Autodesk Inventor part; units mm, degrees
ref_plane "YZ Plane" through (0, 0, 0) normal (1, 0, 0) x (0, 1, 0)
ref_plane "XZ Plane" through (0, 0, 0) normal (0, 1, 0) x (-1, 0, 0)
ref_plane "XY Plane" through (0, 0, 0) normal (0, 0, 1) x (1, 0, 0)
sketch "Sketch3" plane through (0, 0, 0) normal (0, 0, 1) x (1, 0, 0)
  line L0 (26, 0) -> (21.75, 0.3)
  line L1 (26, 0) -> (26, 18)
  line L2 (21.75, 0.3) -> (21.75, 3.3)
  line L3 (21.75, 3.3) -> (15, 3.3)
  line L4 (15, 3.3) -> (15, 18)
  line L5 (15, 18) -> (26, 18)
  line L6 (0, -3.6) -> (0, 21.6)
  point P0 (0, 0)
  dimension "d5" = 26
  dimension "d6" = 21.75
  dimension "d7" = 0.3
  dimension "d8" = 18
  dimension "d9" = 15
  dimension "d10" = 3
revolve "Revolution1" add sketch "Sketch3" angle 360 about axis through (0, -10, 0) along (0, 1, 0)
sketch "Sketch4" plane through (0, 18, 0) normal (0, 1, 0) x (1, 0, 0)
  point P0 (0, 0)
  point P1 (0, 22)
  point P2 (-19.0526, 11)
  point P3 (-19.0526, -11)
  point P4 (0, -22)
  point P5 (19.0526, -11)
  point P6 (19.0526, 11)
  dimension "d12" = 22
  dimension "d15" = 360
hole "Hole1" at (0, 18, -22) at (-19.0526, 18, -11) at (-19.0526, 18, 11) at (0, 18, 22) at (19.0526, 18, 11) at (19.0526, 18, -11) direction (0, -1, 0) diameter 5 end through all both
properties part number "Adapter1"
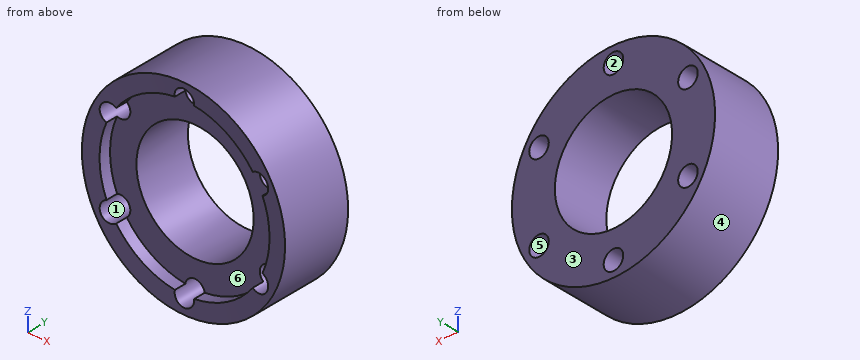
Part model, mm, in its own coordinate system. Face numbers are marked on the shaded views. A direction names the side the tool comes from. Give positions to 0.01 mm unless a question says otherwise; leave off trailing zeros. Order: outer loops, then holes, each group sorted by start corner. A loop starts at its lowest first (then second) coordinate and runs counter-clockwise, first axis right, second up. Notation, with made-up numbers: (-3, 81) - (2, 81) arc R19 cw to (2, 92) - close; hole circle Ø4 at (45, 19.25). An arc over 180 degrees is marked (long way). Use a Markdown table: item, result.
1) Saw through at C-C on x = 0. List the corners of the cut face in (y, z).
Checked values:
| item | result |
|---|---|
| outline | (0, -26) - (18, -26) - (18, -24.5) - (0.11, -24.5) - close; (0, 26) - (0.11, 24.5) - (18, 24.5) - (18, 26) - close; (3.3, -19.5) - (18, -19.5) - (18, -15) - (3.3, -15) - close; (3.3, 15) - (18, 15) - (18, 19.5) - (3.3, 19.5) - close |
2) Saw through at B-B on y = 1.5. List the corners of the cut face in (x, z), plus the area to 3 significant figures.
Checked values:
| item | result |
|---|---|
| outline | circle Ø52 at (0, 0); hole (-19.95, -8.67) arc R2.5 ccw (long way) to (-17.48, -12.94) arc R21.75 ccw to (-2.47, -21.61) arc R2.5 ccw (long way) to (2.47, -21.61) arc R21.75 ccw to (17.48, -12.94) arc R2.5 ccw (long way) to (19.95, -8.67) arc R21.75 ccw to (19.95, 8.67) arc R2.5 ccw (long way) to (17.48, 12.94) arc R21.75 ccw to (2.47, 21.61) arc R2.5 ccw (long way) to (-2.47, 21.61) arc R21.75 ccw to (-17.48, 12.94) arc R2.5 ccw (long way) to (-19.95, 8.67) arc R21.75 ccw to start |
| area | 570 mm² |
3) Saw through at A-A on z = 0. List the corners of the cut face in (x, y), plus the area to 3 significant figures.
Checked values:
| item | result |
|---|---|
| outline | (-26, 0) - (-21.75, 0.3) - (-21.75, 3.3) - (-15, 3.3) - (-15, 18) - (-26, 18) - close; (15, 3.3) - (21.75, 3.3) - (21.75, 0.3) - (26, 0) - (26, 18) - (15, 18) - close |
| area | 350 mm² |
4) Saw through at D-D on y = 11. List the corners of the cut face in (x, z), plus the area to 3 significant figures.
Checked values:
| item | result |
|---|---|
| outline | circle Ø52 at (0, 0); hole circle Ø5 at (-19.05, -11); hole circle Ø5 at (-19.05, 11); hole circle Ø30 at (0, 0); hole circle Ø5 at (0, -22); hole circle Ø5 at (0, 22); hole circle Ø5 at (19.05, -11); hole circle Ø5 at (19.05, 11) |
| area | 1,300 mm² |
5) Probe L1, parallel to Z at x = 18, y = 12.5; L2, parallel to X at y = 4.5, z = 11; L3, parallel to Z at x = 0, y = 12. List the from-to ranges inside material, lowest first. Write a range as from..to.
Checked values:
| item | result |
|---|---|
| L1 | -18.76..-13.27, -8.73..8.73, 13.27..18.76 |
| L2 | -23.56..-21.55, -16.55..-10.2, 10.2..16.55, 21.55..23.56 |
| L3 | -26..-24.5, -19.5..-15, 15..19.5, 24.5..26 |
6) Flat gauge pins, fed straight in: P1, Ø5, axis at x = 15, y = 5.5, coming from the +Z side; P2, Ø10, axis at x = 13.5, y = 16, coming from the -Z side; P3, Ø6, axis at y = 10.5, z = 4.5, coming from the +X side. Where does each tip first touch, or does it go through?
Checked values:
| item | result |
|---|---|
| P1 | z = 22.8 |
| P2 | z = -24.57 |
| P3 | x = 25.96 |
7) Two-plate mould, pull along X, no slides. Class the marked faces 1, 2, 3 and 4: +X half, -X half, draft (parallel to the pull), parting line (faces both ways), or undercut.
Checked values:
| item | result |
|---|---|
| face 1 | undercut |
| face 2 | undercut |
| face 3 | draft |
| face 4 | parting line |
8) 3-axis set-ups, long thin cutter, end or side, ignore diameter. For the marked faces 5 and 6: which of +Z, -Z, +X, -X, +Y, -Y reach the whole face in a straight line?
Checked values:
| item | result |
|---|---|
| face 5 | +Y, -Y |
| face 6 | -Y |
